Work out the finished part from the listing and answer in its coordinate system (mm). A direction names the side the tool comes from. Give positions to 0.01 mm unless a question says otherwise; leave off trailing zeros. Order: outer loops, then holes, each group sorted by start corner. A loop starts at its lowest first (then second) coordinate and runs counter-clockwise, first axis right, second up. Notation, with made-up numbers: (-37.5, 53) -> (-19.5, 53) arc R12 cw to (-19.5, 58) -> close; hole circle Ø10 at (-20, -2). An arc over 180 degrees is marked (long way). Answer as CSV lines item,"result". Start each with the question number.
1. Flat-ended cylindrical pins translate along their axes: pin 1 (8 mm diameter, centred on x = 9.5, y = -8.5, fed in from -Z); pin 2 (4 mm diameter, centred on y = 6, z = -4, fed in from +X); pin 3 (6 mm diameter, centred on y = 8, z = 12.5, fed in from +X). Find the tip coordinate at first contact, or state that the pin passes through.
2. A cutting plane is placed at C-C (z = 6.5). Give the vertices of the cut face in (x, y), then the cut area to 3 significant figures.
3. For a pull along Z with two mould halves and no side action, classify faces 4 (the cylindrical face through (-1.08, -4.88, 13.97)), 5 (the cylindrical face through (-14.985, 0.66, 17.479)), 6 (the flat face through (-0.2, -8.2, 0)) as released by +Z, released by -Z, zero draft, split by the parting line, or undercut.
4. A cutting plane is placed at A-A (y = 0). Give the vertices of the cut face in (x, z), then the cut area to 3 significant figures.
5. Find the intervals of material crossed by L1, parallel to Z at x = -5, y = -6.5; L2, parallel to Z at x = -3, y = 6.25; L3, parallel to Y at x = -6.25, z = -6, in increasing order.
6. A cutting plane is placed at D-D (z = -11.5). Give the vertices of the cut face in (x, y), then the cut area to 3 significant figures.
7. For faces 1 (the flat face through (-0.2, -5.4, 12)), 2 (the cylindrical face through (-1.73, 7.81, -7.4)), 3 (the flat face through (0, 0, 21)), determine the directions among +Z, -Z, +X, -X, +Y, -Y from which every point of the face is accessible in a straight line to the end or side of a thin tool.
from build123d import *

# Parameters (mm, degrees)
F0_R     = 12.5
F1_DEPTH = 12
F2_R     = 8
F3_DEPTH = 15
F4_R     = 5
F5_DEPTH = 4
F6_R     = 15
F6_R_2   = 5
F7_DEPTH = 5
F8_SIZE2 = 2
F8_SIZE  = 6


with BuildPart() as f1:
    # F0 (on Top) → F1 (new body)
    with BuildSketch(Plane.XY):
        Circle(F0_R)
    extrude(amount=F1_DEPTH)

    # F2 (on face) → F3 (join)
    with BuildSketch(Plane(origin=(0, 0, 0), x_dir=(1, 0, 0), z_dir=(0, 0, -1))):
        Circle(F2_R)
    extrude(amount=F3_DEPTH)

    # F4 (on face) → F5 (join)
    with BuildSketch(Plane.XY.offset(12)):
        Circle(F4_R)
    extrude(amount=F5_DEPTH)

    # F6 (on face) → F7 (join)
    with BuildSketch(Plane.XY.offset(16)):
        Circle(F6_R)
        Circle(F6_R_2, mode=Mode.SUBTRACT)
        Circle(F6_R_2)
    extrude(amount=F7_DEPTH)

    # F8
    f8_edges = [f1.edges().sort_by_distance(p)[0] for p in [
        (-15, 0, 21),
    ]]
    f8_side = f1.faces().sort_by_distance((0, 0, 21))[0]
    chamfer(f8_edges, length=F8_SIZE, length2=F8_SIZE2, reference=f8_side)


solid = f1.part
Answer sheet:
1,pin 1,"stops at z = 0"
1,pin 2,"stops at x = 6.93"
1,pin 3,"stops at x = 11.44"
2,outline,"circle Ø25 at (0, 0)"
2,area,"491 mm^2"
3,face 4,"undercut"
3,face 5,"zero draft"
3,face 6,"released by -Z"
4,outline,"(-15, 16) -> (-5, 16) -> (-5, 12) -> (-12.5, 12) -> (-12.5, 0) -> (-8, 0) -> (-8, -15) -> (8, -15) -> (8, 0) -> (12.5, 0) -> (12.5, 12) -> (5, 12) -> (5, 16) -> (15, 16) -> (15, 19) -> (9, 21) -> (-9, 21) -> (-15, 19) -> close"
4,area,"718 mm^2"
5,L1,"z = 0 to 12, 16 to 21"
5,L2,"z = -15 to 12, 16 to 21"
5,L3,"y = -4.99 to 4.99"
6,outline,"circle Ø16 at (0, 0)"
6,area,"201 mm^2"
7,face 1,"none"
7,face 2,"-Z"
7,face 3,"+Z, +X, -X, +Y, -Y"
